from build123d import *

# Parameters (mm, degrees)
F0_R     = 0.762
F1_DEPTH = 3.81
F2_R     = 2.54
F3_DEPTH = 0.635
F4_R     = 1.143
F4_R_2   = 0.762
F5_DEPTH = 0.5588
F6_DEPTH = 0.254


with BuildPart() as f1:
    # F0 (on Top) → F1 (new body)
    with BuildSketch(Plane.XY):
        Circle(F0_R)
    extrude(amount=F1_DEPTH)

    # F2 (on face) → F3 (join)
    with BuildSketch(Plane.XY.offset(3.81)):
        Circle(F2_R)
    extrude(amount=-F3_DEPTH)

    # F4 (on face) → F5 (cut)
    with BuildSketch(Plane(origin=(0, 0, 3.175), x_dir=(1, 0, 0), z_dir=(0, 0, -1))):
        Circle(F4_R)
        Circle(F4_R_2, mode=Mode.SUBTRACT)
    extrude(amount=-F5_DEPTH, mode=Mode.SUBTRACT)

    # F6 (add): a face of the model
    f6_faces = [f1.faces().sort_by_distance(p)[0] for p in [
        (-2.468157951, 0, 3.175),
    ]]
    extrude(f6_faces, amount=F6_DEPTH)


solid = f1.part
Verification items for the finished model (mm, model axes). A direction names the side the tool comes from. Coordinates: 2 decimals unless noted, no trailing zeros. Order: outer loops, then holes, each group sorted by start corner. A loop starts at its lowest first (then second) coordinate and runs counter-clockwise, first axis right, second up. Notation, with made-up numbers: (20, 45) -> (50, 45) arc R29 cw to (50, 77) -> close; hole circle Ø7 at (76, 55.5). An arc over 180 degrees is marked (long way). Use CSV: the item, a comma, the result in double quotes. Start each with the question number.
Q1. Section check C-C, the plane z = 3.15. Record the cut outline in (x, y).
Q2. Draft check along X on faces 3 (the cylindrical face through (-0.248, 1.116, 3.333)), 4 (the cylindrical face through (-0.33, 2.52, 3.37)), 5 (the flat face through (1, -1, 2.921)). Enter one of: +X half, -X half, draft (parallel to the pull), parting line (faces both ways), or undercut.
Q3. Depth check by flat-ended pin: P1, Ø1, axis at y = -0.5, z = 1.5, coming from the -X side. Enter the tip coordinate at first touch or a pass-through.
Q4. Tool access check on faces 1 (the flat face through (0, 0, 0)), 2 (the cylindrical face through (-0.099, -0.756, 1.841)). Record the directions out of +Z, -Z, +X, -X, +Y, -Y that give a thin tool (end or side, any length) a straight path to the whole face; none if there is none.
Q5. Section check D-D, the plane z = 0.6. Record the cut outline in (x, y), and give its area (3 significant figures).
Q6. Thickness scan on line 1 along Y through (x, z) = (0, 3.55); line 2 along Z through (x, y) = (-1.45, -1); line 3 along Y through (x, z) = (-1.3, 3.55). Record the ranges inside material, lowest first.
Q7. Section check A-A, the plane x = 0. Record the cut outline in (y, z).
Returned:
1,outline,"circle Ø5.08 at (0, 0); circle Ø1.52 at (0, 0); hole circle Ø2.29 at (0, 0)"
2,face 3,"undercut"
2,face 4,"parting line"
2,face 5,"draft"
3,P1,"stops at x = -0.76"
4,face 1,"-Z, +X, -X, +Y, -Y"
4,face 2,"-Z"
5,outline,"circle Ø1.52 at (0, 0)"
5,area,"1.82 mm^2"
6,line 1,"y = -2.54 to -1.14, -0.76 to 0.76, 1.14 to 2.54"
6,line 2,"z = 2.92 to 3.81"
6,line 3,"y = -2.18 to 2.18"
7,outline,"(-2.54, 2.92) -> (-1.14, 2.92) -> (-1.14, 3.73) -> (-0.76, 3.73) -> (-0.76, 0) -> (0.76, 0) -> (0.76, 3.73) -> (1.14, 3.73) -> (1.14, 2.92) -> (2.54, 2.92) -> (2.54, 3.81) -> (-2.54, 3.81) -> close"
